Can you work these out from the drawing? Everything is in mm from the part's minimum corner. A direction names the side the tool comes from. Give positions to 0.01 mm unless a question says otherwise; leave off trailing zeros. Write each loop counter-clockwise with the first axis right and the second up, starting at its lowest first coordinate (ties: lowest second). Pieces come first, ordered by that corner, then holes. Notation, with made-up numbers: (29, 29.5) - (85, 29.5) arc R15 ccw to (85, 53.5) - close; hole circle Ø2 at (47.25, 7.5). An arc over 180 degrees is marked (long way). Use a Markdown table: item, result.
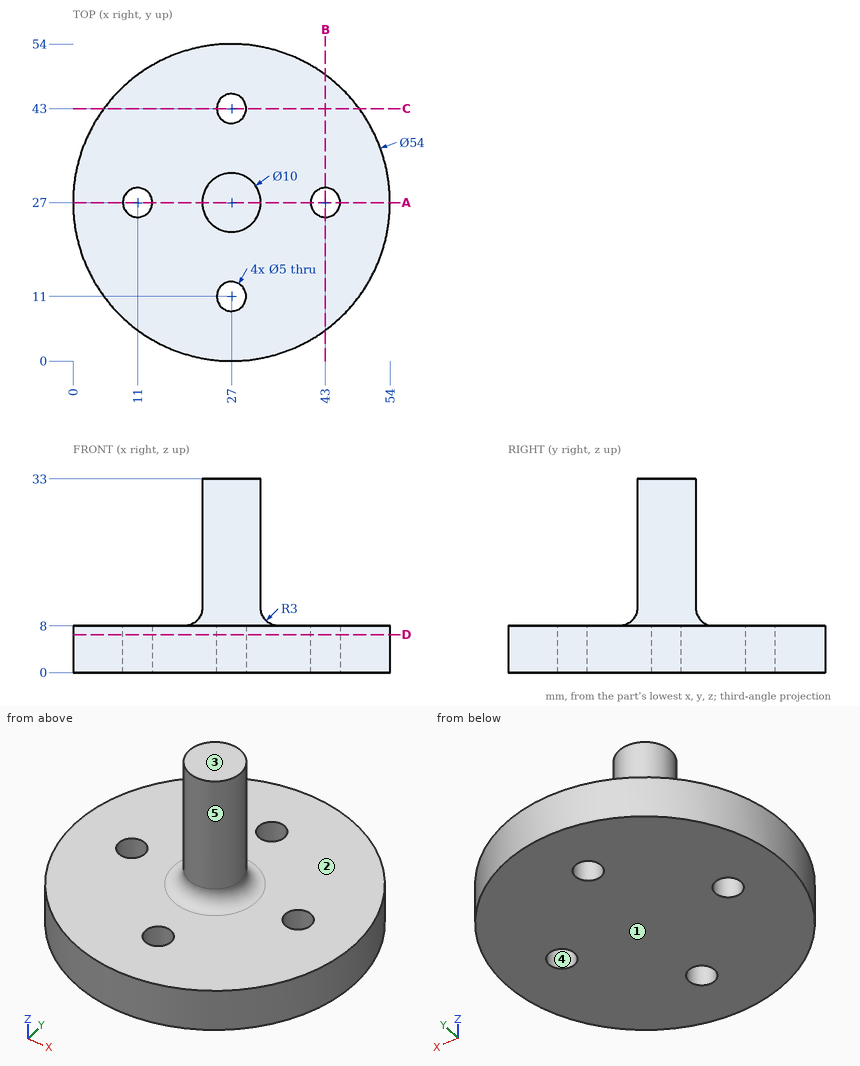
Item 1: I need wall thicknesses on line 1 along Y through (x, z) = (27, 6); line 2 along Z through (x, y) = (43.5, 21); line 3 along Y through (x, z) = (43, 5.75). Which ranges of each line are inside material? Lowest first, please. Write a range as [from, to].
Values:
| item | result |
|---|---|
| line 1 | y = [0, 8.5], [13.5, 40.5], [45.5, 54] |
| line 2 | z = [0, 8] |
| line 3 | y = [5.25, 24.5], [29.5, 48.75] |
Item 2: For the marked faces 1 and 2, which set-ups out of +Z, -Z, +X, -X, +Y, -Y let a thin tool reach every point of the face, with its end or its side?
Values:
| item | result |
|---|---|
| face 1 | -Z, +X, -X, +Y, -Y |
| face 2 | +Z |
Item 3: Thinking about a two-plate mould opening in X: for the marked faces 3, 4 and 5, which applies, +X half, -X half, draft (parallel to the pull), parting line (faces both ways), or undercut?
Values:
| item | result |
|---|---|
| face 3 | draft |
| face 4 | undercut |
| face 5 | parting line |
Item 4: If we section it at A-A, the plane y = 27: Write out the boundary of the cut face in (x, z).
Values:
| item | result |
|---|---|
| outline | (0, 0) - (8.5, 0) - (8.5, 8) - (0, 8) - close; (13.5, 0) - (40.5, 0) - (40.5, 8) - (35, 8) arc R3 cw to (32, 11) - (32, 33) - (22, 33) - (22, 11) arc R3 cw to (19, 8) - (13.5, 8) - close; (45.5, 0) - (54, 0) - (54, 8) - (45.5, 8) - close |
Item 5: If we section it at B-B, the plane x = 43: Write out the boundary of the cut face in (y, z).
Values:
| item | result |
|---|---|
| outline | (5.25, 0) - (24.5, 0) - (24.5, 8) - (5.25, 8) - close; (29.5, 0) - (48.75, 0) - (48.75, 8) - (29.5, 8) - close |
Item 6: If we section it at D-D, the plane z = 6.5: Write out the boundary of the cut face in (x, y), plus the area to 3 significant figures.
Values:
| item | result |
|---|---|
| outline | circle Ø54 at (27, 27); hole circle Ø5 at (11, 27); hole circle Ø5 at (27, 11); hole circle Ø5 at (27, 43); hole circle Ø5 at (43, 27) |
| area | 2,210 mm2 |
Item 7: Will these pins go through, and if not, where does the flat tip stop? pin 1 Ø6 at (x, y) = (27, 43) entering from +Z; pin 2 Ø2 at (y, z) = (24.5, 18.5) entering from -X; pin 3 Ø12 at (x, z) = (44, 17.5) entering from +Y; pin 4 Ø5 at (y, z) = (41.5, 9.5) entering from -X.
Values:
| item | result |
|---|---|
| pin 1 | stops at z = 8 |
| pin 2 | stops at x = 22.23 |
| pin 3 | passes through |
| pin 4 | stops at x = 3.07 |
